The model under review builds one solid part; all positions refer to its coordinate system, in mm. A direction names the side the tool comes from. Give positions to 0.01 mm unless a question says otherwise; leave off trailing zeros. Order: outer loops, then holes, each group sorted by start corner. A loop starts at its lowest first (then second) coordinate and runs counter-clockwise, first axis right, second up. Notation, with made-up numbers: (48, 52) -> (52, 52) arc R19 ccw to (52, 73) -> close; hole circle Ø5 at (49, -19). An arc over 180 degrees is marked (long way). Answer as a JSON object with one key per item and string values. Group by question number.
from build123d import *

# Parameters (mm, degrees)
SKETCH_1_W          = 99
SKETCH_1_H          = 104
SKETCH_1_R          = 1.5
SKETCH_1_W_2        = 95
SKETCH_1_H_2        = 61
EXTRUDE_3_DEPTH     = 3
SKETCH_3_W          = 99
SKETCH_3_H          = 104
SKETCH_3_W_2        = 95
SKETCH_3_H_2        = 100
EXTRUDE_4_DEPTH     = 33
CUT_EXTRUDE_2_DEPTH = 30
SKETCH_5_W          = 60
SKETCH_5_H          = 7.5
CUT_EXTRUDE_3_DEPTH = 30
SKETCH_6_W          = 28
SKETCH_6_H          = 55
CUT_EXTRUDE_4_DEPTH = 30
SKETCH_7_W          = 7.5
SKETCH_7_H          = 20
CUT_EXTRUDE_5_DEPTH = 30
SKETCH_8_W          = 23.5
SKETCH_8_H          = 7.5
CUT_EXTRUDE_6_DEPTH = 30
FILLET_1_R          = 1


with BuildPart() as part:
    # 草图1 → 凸台-拉伸3 (new body)
    with BuildSketch(Plane.XY):
        with Locations((0, -11.5)):
            Rectangle(SKETCH_1_W, SKETCH_1_H)
        with Locations((43, 34)):
            Circle(SKETCH_1_R, mode=Mode.SUBTRACT)
        with Locations(Location((-44.813801575, 34, 0), (0, 0, 180))):
            Circle(SKETCH_1_R, mode=Mode.SUBTRACT)
        with Locations((-44.813801575, -34)):
            Circle(SKETCH_1_R, mode=Mode.SUBTRACT)
        with Locations(Location((43, -34, 0), (0, 0, 180))):
            Circle(SKETCH_1_R, mode=Mode.SUBTRACT)
        Rectangle(SKETCH_1_W_2, SKETCH_1_H_2, mode=Mode.SUBTRACT)
    extrude(amount=EXTRUDE_3_DEPTH)

    # 草图3 → 凸台-拉伸4 (add)
    with BuildSketch(Plane.XY.offset(3)):
        with Locations((0, -11.5)):
            Rectangle(SKETCH_3_W, SKETCH_3_H)
        with Locations((0, -11.5)):
            Rectangle(SKETCH_3_W_2, SKETCH_3_H_2, mode=Mode.SUBTRACT)
    extrude(amount=EXTRUDE_4_DEPTH)

    # 草图4 → 切除-拉伸2 (cut)
    with BuildSketch(Plane.ZY.offset(-47.5)):
        Polygon((3, 30.5), (12, 30.5), (12, -30.5), (3, -30.5), (0, -30.5), (0, 30.5), align=None)
    extrude(amount=-CUT_EXTRUDE_2_DEPTH, mode=Mode.SUBTRACT)

    # 草图5 → 切除-拉伸3 (cut)
    with BuildSketch(Plane(origin=(0, 40.5, 0), x_dir=(1, 0, 0), z_dir=(0, 1, 0))):
        with Locations((-17.5, -24.75)):
            Rectangle(SKETCH_5_W, SKETCH_5_H)
    extrude(amount=-CUT_EXTRUDE_3_DEPTH, mode=Mode.SUBTRACT)

    # 草图6 → 切除-拉伸4 (cut)
    with BuildSketch(Plane.ZY.offset(-47.5)):
        with Locations((22, 11)):
            Rectangle(SKETCH_6_W, SKETCH_6_H)
    extrude(amount=-CUT_EXTRUDE_4_DEPTH, mode=Mode.SUBTRACT)

    # 草图7 → 切除-拉伸5 (cut)
    with BuildSketch(Plane.ZY.offset(-47.5)):
        with Locations((24.75, -41.5)):
            Rectangle(SKETCH_7_W, SKETCH_7_H)
    extrude(amount=-CUT_EXTRUDE_5_DEPTH, mode=Mode.SUBTRACT)

    # 草图8 → 切除-拉伸6 (cut)
    with BuildSketch(Plane(origin=(0, -61.5, 0), x_dir=(1, 0, 0), z_dir=(0, 1, 0))):
        with Locations((28.25, -24.75)):
            Rectangle(SKETCH_8_W, SKETCH_8_H)
    extrude(amount=-CUT_EXTRUDE_6_DEPTH, mode=Mode.SUBTRACT)

    # 圆角1
    fillet_1_edges = [part.edges().sort_by_distance(p)[0] for p in [
        (-49.5, 40.5, 18),
        (49.5, 40.5, 18),
        (49.5, -63.5, 18),
        (-49.5, -63.5, 18),
    ]]
    fillet(fillet_1_edges, radius=FILLET_1_R)


solid = part.part
1. For probe 1 along Y at (x, z) = (43, 1.7); probe 2 along Y at (x, z) = (-23, 5); probe 3 along X at (y, z) = (-35, 17.5), list the stretches that pass through material, from the lowest coordinate up. Write a range as [from, to].
2. Take a section at A-A on y = -46.5. Give the boundary of the cut face in (x, z), plus the area to 3 significant figures.
3. Draft analysis for pull direction X (two halves, no side actions). For faces 3 (the flat face through (-1, -34, 0)), 4 (the flat face through (-49.5, -12, 18)), 5 (the flat face through (47.5, -39, 19)), state which applies: pulls with the +X half, pulls with the -X half, needs draft (parallel to the pull), parting line crosses it, or undercut.
4. Take a section at B-B on x = 43. Give the boundary of the cut face in (y, z), plus the area to 3 significant figures.
5. For pin 1 (1.5 mm diameter, centred on y = -14, z = 25.5, fed in from +X); pin 2 (1.5 mm diameter, centred on x = -4, z = 27, fed in from +Y); pin 3 (1 mm diameter, centred on x = 48, y = 32.5, fed in from +Z), all flat-tipped, find the tip position at first contact; note any pin that passes through.
6. Take a section at C-C on z = 25. Give the boundary of the cut face in (x, y), plus the area to 3 significant figures.
7. Machinability: for faces 1 (the flat face through (-48, 12, 36)), 2 (the flat face through (-1, 35, 3)), which of the approach directions +Z, -Z, +X, -X, +Y, -Y give a long, thin tool a straight path to every point of the face, cutting with its end or side? Answer none if there is none.
8. Take a section at D-D on x = -29.5. Give the boundary of the cut face in (y, z), plus the area to 3 significant figures.
Checks:
{
 "1": {"probe 1": "y = [-63.5, -35.5], [-32.5, -30.5], [30.5, 32.5], [35.5, 40.5]", "probe 2": "y = [-63.5, -61.5], [38.5, 40.5]", "probe 3": "x = [-49.5, -47.5], [47.5, 49.5]"},
 "2": {"outline": "(-49.5, 0) -> (49.5, 0) -> (49.5, 21) -> (47.5, 21) -> (47.5, 3) -> (-47.5, 3) -> (-47.5, 36) -> (-49.5, 36) -> close; (47.5, 28.5) -> (49.5, 28.5) -> (49.5, 36) -> (47.5, 36) -> close", "area": "414 mm2"},
 "3": {"face 3": "needs draft", "face 4": "pulls with the -X half", "face 5": "undercut"},
 "4": {"outline": "(-63.5, 0) -> (-35.5, 0) -> (-35.5, 3) -> (-61.5, 3) -> (-61.5, 36) -> (-63.5, 36) -> close; (-32.5, 0) -> (-30.5, 0) -> (-30.5, 3) -> (-32.5, 3) -> close; (30.5, 0) -> (32.5, 0) -> (32.5, 3) -> (30.5, 3) -> close; (35.5, 0) -> (40.5, 0) -> (40.5, 36) -> (38.5, 36) -> (38.5, 3) -> (35.5, 3) -> close", "area": "243 mm2"},
 "5": {"pin 1": "stops at x = -47.5", "pin 2": "stops at y = -61.5", "pin 3": "stops at z = 8"},
 "6": {"outline": "(-49.5, -62.5) arc R1 ccw to (-48.5, -63.5) -> (16.5, -63.5) -> (16.5, -61.5) -> (-47.5, -61.5) -> (-47.5, 40.5) -> (-48.5, 40.5) arc R1 ccw to (-49.5, 39.5) -> close; (12.5, 38.5) -> (49.5, 38.5) -> (49.5, 39.5) arc R1 ccw to (48.5, 40.5) -> (12.5, 40.5) -> close; (40, -63.5) -> (48.5, -63.5) arc R1 ccw to (49.5, -62.5) -> (49.5, -51.5) -> (47.5, -51.5) -> (47.5, -61.5) -> (40, -61.5) -> close; (47.5, -31.5) -> (49.5, -31.5) -> (49.5, -16.5) -> (47.5, -16.5) -> close", "area": "478 mm2"},
 "7": {"face 1": "+Z, +X, -X, +Y, -Y", "face 2": "+Z"},
 "8": {"outline": "(-63.5, 0) -> (-30.5, 0) -> (-30.5, 3) -> (-61.5, 3) -> (-61.5, 36) -> (-63.5, 36) -> close; (30.5, 0) -> (40.5, 0) -> (40.5, 21) -> (38.5, 21) -> (38.5, 3) -> (30.5, 3) -> close; (38.5, 28.5) -> (40.5, 28.5) -> (40.5, 36) -> (38.5, 36) -> close", "area": "246 mm2"}
}
